The listing builds one solid part. Answer for the finished solid, in the listing's coordinates (mm). A direction names the side the tool comes from. Coordinates: 2 decimals unless noted, no trailing zeros. Order: outer loops, then holes, each group sorted by start corner. A loop starts at its lowest first (then second) coordinate and runs counter-clockwise, first axis right, second up.
```python
from build123d import *

# Parameters (mm, degrees)
BOSS_EXTRUDE1_DEPTH            = 9.525
F_7_0_201_DIAMETER_SLOT1_DEPTH = 9.525
FILLET1_R                      = 3.175


# Read off the part's stored shape, not the designer's step: #7 (0.201) Diameter Slot1
with BuildPart() as part:
    # Sketch1 → Boss-Extrude1 (new body)
    with BuildSketch(Plane(origin=(0, 0, 0), x_dir=(1, 0, 0), z_dir=(0, 1, 0))):
        with BuildLine():
            Line((0, 0), (304.8, 0))
            Line((304.8, 0), (304.8, 122.2375))
            Line((304.8, 122.2375), (241.3, 122.2375))
            ThreePointArc((241.3, 122.2375), (214.3125, 149.225), (241.3, 176.2125))
            Line((241.3, 176.2125), (304.8, 176.2125))
            Line((304.8, 176.2125), (304.8, 228.6))
            Line((304.8, 228.6), (193.694523922, 228.6))
            Line((193.694523922, 228.6), (96.847261961, 177.8))
            Line((96.847261961, 177.8), (0, 177.8))
            Line((0, 177.8), (0, 136.525))
            Line((0, 136.525), (193.694523922, 136.525))
            Line((193.694523922, 136.525), (193.694523922, 41.275))
            Line((193.694523922, 41.275), (0, 41.275))
            Line((0, 41.275), (0, 0))
        make_face()
    extrude(amount=BOSS_EXTRUDE1_DEPTH)

    # #7 (0.201) Diameter Slot1 outline → #7 (0.201) Diameter Slot1 (cut)
    with BuildSketch(Plane(origin=(0, 0, 0), x_dir=(1, 0, 0), z_dir=(0, 1, 0))):
        with BuildLine():
            Line((8.922223922, 151.076161), (22.866823922, 151.076161))
            ThreePointArc((22.866823922, 151.076161), (25.419523922, 153.628861), (22.866823922, 156.181561))
            Line((22.866823922, 156.181561), (8.922223922, 156.181561))
            ThreePointArc((8.922223922, 156.181561), (6.369523922, 153.628861), (8.922223922, 151.076161))
        make_face()
        with BuildLine():
            ThreePointArc((124.466823922, 151.076161), (127.019523922, 153.628861), (124.466823922, 156.181561))
            Line((124.466823922, 156.181561), (110.522223922, 156.181561))
            ThreePointArc((110.522223922, 156.181561), (107.969523922, 153.628861), (110.522223922, 151.076161))
            Line((110.522223922, 151.076161), (124.466823922, 151.076161))
        make_face()
        with BuildLine():
            Line((8.922223922, 21.618439), (22.866823922, 21.618439))
            ThreePointArc((22.866823922, 21.618439), (25.419523922, 24.171139), (22.866823922, 26.723839))
            Line((22.866823922, 26.723839), (8.922223922, 26.723839))
            ThreePointArc((8.922223922, 26.723839), (6.369523922, 24.171139), (8.922223922, 21.618439))
        make_face()
        with BuildLine():
            ThreePointArc((124.466823922, 21.618439), (127.019523922, 24.171139), (124.466823922, 26.723839))
            Line((124.466823922, 26.723839), (110.522223922, 26.723839))
            ThreePointArc((110.522223922, 26.723839), (107.969523922, 24.171139), (110.522223922, 21.618439))
            Line((110.522223922, 21.618439), (124.466823922, 21.618439))
        make_face()
    extrude(amount=F_7_0_201_DIAMETER_SLOT1_DEPTH, mode=Mode.SUBTRACT)

    # Fillet1
    fillet1_edges = [part.edges().sort_by_distance(p)[0] for p in [
        (0, 4.7625, -41.275),
        (193.694523922, 4.7625, -41.275),
        (193.694523922, 4.7625, -136.525),
        (0, 4.7625, -136.525),
        (0, 4.7625, -177.8),
        (96.847261961, 4.7625, -177.8),
        (193.694523922, 4.7625, -228.6),
        (304.8, 4.7625, -228.6),
        (304.8, 4.7625, -176.2125),
        (304.8, 4.7625, -122.2375),
        (304.8, 4.7625, 0),
        (0, 4.7625, 0),
    ]]
    fillet(fillet1_edges, radius=FILLET1_R)


solid = part.part
```
(1) Find section D-D (z = -79). Write down the section's boundary in (x, y) (3 decimals).
(2) The mould has two halves that part along Z. Classify faces 5 (the face through (117, 5, -21.618)), 6 (the face through (304.8, 5, -60)), 7 (the face through (50, 5, -177.8)): released by +Z, released by -Z, zero draft, split by the parting line, or undercut.
(3) Find section C-C (x = 75.5). Write down the section's boundary in (y, z) (3 decimals), and give its area (3 significant figures).
(4) Consider line 1 (Z direction, x = 16, y = 3) (3 decimals); line 2 (Z direction, x = 35.5, y = 1) (3 decimals); line 3 (Z direction, x = 275.5, y = 6). Determine where each line is inside the solid, lowest interval first.
(5) Each of these flat-tipped pins is pushed along its axis until it touches: pin 1 Ø2 at (x, y) = (183, 7.5) entering from -Z; pin 2 Ø5 at (x, y) = (95, 5.5) entering from -Z; pin 3 Ø5 at (x, y) = (53, 5.5) entering from -Z. Where does it stop, or does it pass through?
(6) For faces 1 (the face through (193.695, 5, -90)), 2 (the face through (272, 5, -122.238)), 3 (the face through (0, 5, -21)), 4 (the face through (117, 5, -151.076)), determine the directions among +Z, -Z, +X, -X, +Y, -Y from which every point of the face is accessible in a straight line to the end or side of a thin tool.
(7) Find section B-B (y = 5.25). Give the number of separate pieces and of enclosed holes in the cut face, and give its area (3 significant figures).
(8) Find section A-A (x = 276.5). Write down the section's boundary in (y, z) (1 decimal), and give its area (3 significant figures).
Findings below:
1. outline: (193.695, 0) - (304.8, 0) - (304.8, 9.525) - (193.695, 9.525) - close
2. face 5: undercut
2. face 6: zero draft
2. face 7: released by -Z
3. outline: (0, -177.8) - (9.525, -177.8) - (9.525, -136.525) - (0, -136.525) - close; (0, -41.275) - (9.525, -41.275) - (9.525, 0) - (0, 0) - close
3. area: 786 mm2
4. line 1: z = -177.8 to -156.182, -151.076 to -136.525, -41.275 to -26.724, -21.618 to 0
4. line 2: z = -177.8 to -136.525, -41.275 to 0
4. line 3: z = -228.6 to -176.21, -122.24 to 0
5. pin 1: stops at z = -223.51
5. pin 2: stops at z = -178.14
5. pin 3: stops at z = -177.8
6. face 1: -X, +Y, -Y
6. face 2: +X, +Y, -Y
6. face 3: +Z, -Z, -X, +Y, -Y
6. face 4: +Y, -Y
7. separate pieces: 1
7. enclosed holes: 4
7. area: 38,900 mm2
8. outline: (0, -228.6) - (9.5, -228.6) - (9.5, -176.2) - (0, -176.2) - close; (0, -122.2) - (9.5, -122.2) - (9.5, 0) - (0, 0) - close
8. area: 1,660 mm2
